Verification items for this drawing (mm, ordinates from the low corner). A direction names the side the tool comes from. Round coordinates to 2 decimals unless told otherwise and drop trailing zeros. Loops run counter-clockwise (first coordinate to the right, second up) from the corner with the lowest first, then second, coordinate; pieces in that order, holes last. Notation, with made-up numbers: (14, 23.25) - (72, 23.25) arc R30 ccw to (72, 62.25) - close; hole circle Ø3 at (55.5, -27.75). An arc over 180 degrees is marked (long way). Put each result on its own line as item: value.
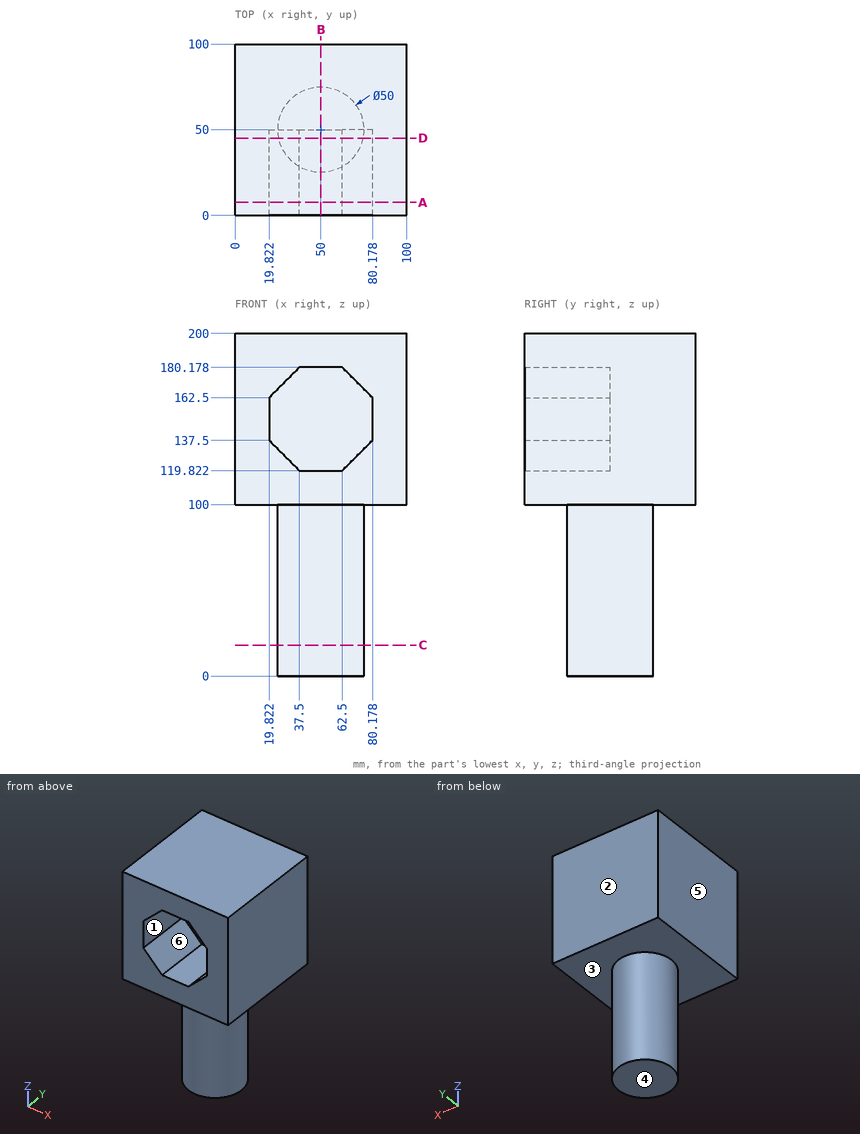
Item 1: Section check D-D on y = 45. Enter the section's corners in (x, z) (1 decimal).
Filled sheet:
outline: (0, 100) - (25.5, 100) - (25.5, 0) - (74.5, 0) - (74.5, 100) - (100, 100) - (100, 200) - (0, 200) - close; hole (19.8, 137.5) - (37.5, 119.8) - (62.5, 119.8) - (80.2, 137.5) - (80.2, 162.5) - (62.5, 180.2) - (37.5, 180.2) - (19.8, 162.5) - close
Item 2: Tool access check on the marked faces 1, 2 and 3. Record the directions out of +Z, -Z, +X, -X, +Y, -Y that give a thin tool (end or side, any length) a straight path to the whole face; none if there is none.
Filled sheet:
face 1: -Y
face 2: +Z, -Z, +X, -X, +Y
face 3: -Z
Item 3: Thickness scan on line 1 (X direction, y = 30, z = 146); line 2 (Z direction, x = 50, y = 18); line 3 (Z direction, x = 5.5, y = 8). Record the ranges inside material, lowest first. Write a range as from..to.
Filled sheet:
line 1: 0..19.82, 80.18..100
line 2: 100..119.82, 180.18..200
line 3: 100..200
Item 4: Release check for a two-part mould opening along X. For the marked faces 4, 5 and 6 record: +X half, -X half, draft (parallel to the pull), parting line (faces both ways), or undercut.
Filled sheet:
face 4: draft
face 5: -X half
face 6: undercut
Item 5: Section check C-C on z = 18. Enter the section's corners in (x, y), then the cut area to 3 significant figures.
Filled sheet:
outline: circle Ø50 at (50, 50)
area: 1,960 mm²
Item 6: Section check B-B on x = 50. Enter the section's corners in (y, z).
Filled sheet:
outline: (0, 100) - (25, 100) - (25, 0) - (75, 0) - (75, 100) - (100, 100) - (100, 200) - (0, 200) - (0, 180.18) - (50, 180.18) - (50, 119.82) - (0, 119.82) - close
Item 7: Go/stop test with flat-tipped pins: pin 1 (12.5 mm diameter, centred on x = 44, y = 32.5, fed in from -Z); pin 2 (8 mm diameter, centred on x = 15, y = 13.5, fed in from -Z); pin 3 (10 mm diameter, centred on x = 22, z = 78.5, fed in from -Y). Record where each tip stops, or that it passes through.
Filled sheet:
pin 1: z = 0
pin 2: z = 100
pin 3: y = 40.2
Item 8: Section check A-A on y = 7.5. Enter the section's corners in (x, z), then the cut area to 3 significant figures.
Filled sheet:
outline: (0, 100) - (100, 100) - (100, 200) - (0, 200) - close; hole (19.82, 137.5) - (37.5, 119.82) - (62.5, 119.82) - (80.18, 137.5) - (80.18, 162.5) - (62.5, 180.18) - (37.5, 180.18) - (19.82, 162.5) - close
area: 6,980 mm²
